Build history of the part. All positions in model axes, mm. Coordinates: 2 decimals unless noted, no trailing zeros. Loops run counter-clockwise (first coordinate to the right, second up) from the corner with the lowest first, then second, coordinate; pieces in that order, holes last.
(1) Flat gauge pins, fed straight in: P1, Ø5.5, axis at x = -9.525, z = 63.5, coming from the -Y side; P2, Ø8, axis at x = 27.305, z = 63.5, coming from the -Y side. Where does each tip first touch, or does it go through?
(2) Slice it at A-A (z = 63.5). Give the cut face in (x, y) (3 decimals), and give its area (3 significant figures).
(3) Wall check: L1, parallel to X at y = 4.75, z = 63.5 (3 decimals). Give the ranges that are in metal, low to high.
from build123d import *

# Parameters (mm, degrees)
SKETCH1_W           = 374.65
SKETCH1_H           = 17.78
BOSS_EXTRUDE1_DEPTH = 127
SKETCH2_R           = 3.556
CUT_EXTRUDE1_DEPTH  = 228.014942295


with BuildPart() as part:
    # Sketch1 → Boss-Extrude1 (new body)
    with BuildSketch(Plane.XY):
        Rectangle(SKETCH1_W, SKETCH1_H)
    extrude(amount=BOSS_EXTRUDE1_DEPTH)

    # Sketch2 → Cut-Extrude1 (cut, through all)
    with BuildSketch(Plane.XZ.offset(8.89)):
        with Locations(Location((-9.525, 63.5, 0), (0, 0, 270))):
            Circle(SKETCH2_R)
        with Locations(Location((27.305, 63.5, 0), (0, 0, 270))):
            Circle(SKETCH2_R)
    extrude(amount=-CUT_EXTRUDE1_DEPTH, mode=Mode.SUBTRACT)


solid = part.part
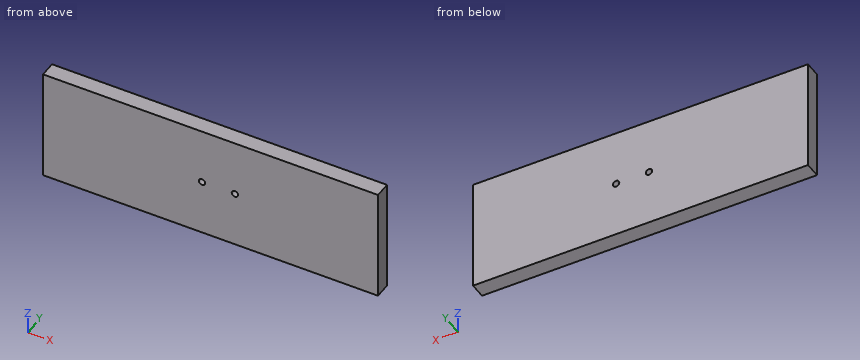
Response values:
1. P1: passes through
1. P2: stops at y = -8.89
2. outline: (-187.325, -8.89) - (-13.081, -8.89) - (-13.081, 8.89) - (-187.325, 8.89) - close; (-5.969, -8.89) - (23.749, -8.89) - (23.749, 8.89) - (-5.969, 8.89) - close; (30.861, -8.89) - (187.325, -8.89) - (187.325, 8.89) - (30.861, 8.89) - close
2. area: 6,410 mm2
3. L1: x = -187.325 to -13.081, -5.969 to 23.749, 30.861 to 187.325
